Autodesk Inventor part; units mm, degrees
ref_plane "YZ Plane" through (0, 0, 0) normal (1, 0, 0) x (0, 1, 0)
ref_plane "XZ Plane" through (0, 0, 0) normal (0, 1, 0) x (-1, 0, 0)
ref_plane "XY Plane" through (0, 0, 0) normal (0, 0, 1) x (1, 0, 0)
sketch "草圖1" plane through (0, 0, 0) normal (0, 1, 0) x (-1, 0, 0)
  line L0 (0, 0) -> (-50, 0)
  line L1 (-50, 0) -> (-50, -40)
  line L2 (-50, -40) -> (0, -40)
  line L3 (0, -40) -> (0, 0)
  dimension "d0" = 50
  dimension "d1" = 40
extrude "擠出1" add sketch "草圖1" along normal blind 20
sketch "草圖2" plane through (0, 20, 0) normal (0, 1, 0) x (1, 0, 0)
  line L0 (50, 40) -> (0, 40)
  line L1 (0, 0) -> (50, 0)
  line L2 (0, 40) -> (30, 40)
  line L3 (30, 40) -> (30, 0)
  line L4 (30, 0) -> (0, 0)
  line L5 (0, 0) -> (0, 40)
  dimension "d4" = 30
extrude "擠出2" add sketch "草圖2" along normal blind 20
fillet "圓角1" radius 20 2 edges at (0, 20, 0) (0, 20, -40)
sketch "草圖3" plane through (0, 40, 0) normal (0, 1, 0) x (1, 0, 0)
  arc A0 (20, 40) -> (20, 0) centre (20, 20) ccw
  line L0 (20, 0) -> (30, 0)
  line L1 (30, 0) -> (30, 40)
  line L2 (30, 40) -> (20, 40)
  arc A1 (20, 30) -> (20, 10) centre (20, 20) ccw
  line L3 (20, 30) -> (20, 30)
  line L4 (20, 30) -> (20, 10)
  line L5 (20, 10) -> (20, 10)
  line L6 (20, 30) -> (39.9509, 30)
  line L7 (39.9509, 30) -> (39.9509, 10)
  line L8 (39.9509, 10) -> (20, 10)
  line L9 (20, 10) -> (20, 30)
  point P0 (0, 0)
  dimension "d8" = 20
extrude "擠出3" cut sketch "草圖3" against normal blind 20 contours L6 L7 L8 L1 | L1 L8 L4 L6 | L4 A1
sketch "草圖4" plane through (0, 20, 0) normal (0, 1, 0) x (1, 0, 0)
  line L0 (50, 0) -> (50, 40)
  circle A0 centre (50, 20) radius 10
  point P0 (0, 0)
  dimension "d11" = 20
extrude "擠出4" cut sketch "草圖4" against normal blind 20
properties part number "29"
Work out the finished part from the listing and answer in its coordinate system (mm). A direction names the side the tool comes from. Round coordinates to 2 decimals unless told otherwise and drop trailing zeros. Write each loop counter-clockwise with the first axis right and the second up, starting at its lowest first coordinate (ties: lowest second). Pieces come first, ordered by that corner, then holes. Notation, with made-up numbers: (25, 73) - (44, 73) arc R16 ccw to (44, 77) - close; hole circle Ø9 at (-9.5, 69.5). An arc over 180 degrees is marked (long way). Return JSON: item names as keys, results as strings. Group by question number.
Q1. The mould has two halves that part along Z. Classify faces 4 (the flat face through (32, 15, -40)), 5 (the flat face through (30, 30, -5)), 6 (the flat face through (30, 20, -20)), 7 (the flat face through (31, 15, 0)): released by +Z, released by -Z, zero draft, split by the parting line, or undercut.
Q2. Each of these flat-tipped pins is pushed along its axis until it touches: pin 1 Ø5 at (x, y) = (9.5, 35) entering from -Z; pin 2 Ø2 at (y, z) = (34, -13.5) entering from +X; pin 3 Ø8 at (y, z) = (32, -5) entering from +X. Where does it stop, or does it pass through?
Q3. The part is cut by section A-A on x = 45. Write down the section's boundary in (y, z).
Q4. The part is cut by section C-C on x = 22.5. Write down the section's boundary in (y, z), then the cut area to 3 significant figures.
Q5. The part is cut by section D-D on z = -29. Write down the section's boundary in (x, y), then the cut area to 3 significant figures.
Q6. Find the intervals of material crossed by L1, parallel to Z at x = 29, y = 28.5; L2, parallel to Y at x = 41, z = -30.5; L3, parallel to X at y = 34, z = -27.5, in increasing order.
Q7. For faces 1 (the flat face through (25, 30, -10)), 2 (the flat face through (25, 0, -20)), 3 (the flat face through (30, 30, -35)), determine the directions among +Z, -Z, +X, -X, +Y, -Y from which every point of the face is accessible in a straight line to the end or side of a thin tool.
Solved:
{
 "1": {"face 4": "released by -Z", "face 5": "zero draft", "face 6": "undercut", "face 7": "released by +Z"},
 "2": {"pin 1": "z = -38.33", "pin 2": "x = 13.39", "pin 3": "x = 30"},
 "3": {"outline": "(0, -40) - (20, -40) - (20, -28.66) - (0, -28.66) - close; (0, -11.34) - (20, -11.34) - (20, 0) - (0, 0) - close"},
 "4": {"outline": "(0, -40) - (40, -40) - (40, -30) - (20, -30) - (20, -10) - (40, -10) - (40, 0) - (0, 0) - close", "area": "1,200 mm²"},
 "5": {"outline": "(2.14, 0) - (45.64, 0) - (45.64, 20) - (15.64, 20) - (15.64, 40) - (2.14, 40) - close", "area": "1,140 mm²"},
 "6": {"L1": "-40 to -30, -10 to 0", "L2": "0 to 20", "L3": "1.46 to 13.39"},
 "7": {"face 1": "+X, +Y", "face 2": "+Z, -Z, +X, -X, -Y", "face 3": "+Z, -Z, +X, +Y"}
}
